```python
from build123d import *

# Parameters (mm, degrees)
BOSS_EXTRUDE1_DEPTH = 3.175
FILLET1_R           = 2
FILLET2_R           = 2
FILLET3_R           = 2


with BuildPart() as part:
    # Sketch2 → Boss-Extrude1 (new body)
    with BuildSketch(Plane(origin=(0, 0, 0), x_dir=(1, 0, 0), z_dir=(0, 1, 0))):
        with BuildLine():
            Line((0, 0), (40, 0))
            Line((40, 0), (40, 10))
            ThreePointArc((40, 10), (32.396249588, 7.141230333), (25, 10.500557105))
            Line((25, 10.500557105), (25, 20.002146828))
            Line((25, 20.002146828), (24.05, 20.002146828))
            Line((24.05, 20.002146828), (24.05, 5.002146828))
            Line((24.05, 5.002146828), (15.95, 5.002146828))
            Line((15.95, 5.002146828), (15.95, 20.002146828))
            Line((15.95, 20.002146828), (15, 20.002146828))
            Line((15, 20.002146828), (15, 9.499442895))
            ThreePointArc((15, 9.499442895), (7.396249588, 6.640673228), (0, 10))
            Line((0, 10), (0, 0))
        make_face()
    extrude(amount=BOSS_EXTRUDE1_DEPTH)

    # Fillet1
    fillet1_edges = [part.edges().sort_by_distance(p)[0] for p in [
        (15, 1.5875, -9.499442895),
        (25, 1.5875, -10.500557105),
    ]]
    fillet(fillet1_edges, radius=FILLET1_R)

    # Fillet2
    # the kernel refuses this fillet: 2 mm, written as the material it takes off along each edge
    with BuildSketch(Plane(origin=(25, -4.255511133, -20.002146828), x_dir=(0, 0, 1), z_dir=(0, 1, 0))) as fillet2_piece_1:
        with BuildLine():
            CenterArc((1.702204453, -2), FILLET2_R, 90, 58.331756746)
            Line((0, -0.95), (-0.034044089, -0.929))
            ThreePointArc((-0.034044089, -0.929), (-0.04, -0.475), (-0.04, 0))
            Line((-0.04, 0), (0, 0.04))
            Line((0, 0.04), (1.702204453, 0.04))
            Line((1.702204453, 0.04), (1.702204453, 0))
        make_face()
    extrude(amount=11.686022265, mode=Mode.SUBTRACT)
    with BuildSketch(Plane(origin=(15, -4.255511133, -20.002146828), x_dir=(0, 0, 1), z_dir=(0, 1, 0))) as fillet2_piece_2:
        with BuildLine():
            CenterArc((1.702204453, 2), FILLET2_R, 211.668243254, 58.331756746)
            Line((0, 0.95), (-0.034044089, 0.929))
            ThreePointArc((-0.034044089, 0.929), (-0.04, 0.475), (-0.04, 0))
            Line((-0.04, 0), (0, -0.04))
            Line((0, -0.04), (1.702204453, -0.04))
            Line((1.702204453, -0.04), (1.702204453, 0))
        make_face()
    extrude(amount=11.686022265, mode=Mode.SUBTRACT)
    with BuildSketch(Plane(origin=(0, -9.943835684, -10), x_dir=(0, 0, 1), z_dir=(0, 1, 0))) as fillet2_piece_3:
        with BuildLine():
            CenterArc((3.977534274, 2), FILLET2_R, 152.863608887, 117.136391113)
            Line((2.197687698, 2.912220459), (2.162090766, 2.930464868))
            ThreePointArc((2.162090766, 2.930464868), (1.193071422, 1.385002021), (-0.027308932, 0.02922708))
            Line((-0.027308932, 0.02922708), (0, -0.04))
            Line((0, -0.04), (3.977534274, -0.04))
            Line((3.977534274, -0.04), (3.977534274, 0))
        make_face()
    extrude(amount=23.062671369, mode=Mode.SUBTRACT)
    with BuildSketch(Plane(origin=(40, -9.298695448, -10), x_dir=(-0.8303470474110474, 0, 0.5572466068588987), z_dir=(0, 1, 0))) as fillet2_piece_4:
        with BuildLine():
            CenterArc((3.733360689, 1.97396451), FILLET2_R, 146.134404681, 114.610566722)
            Line((2.072666595, 3.088457724), (2.039452713, 3.110747588))
            Line((2.039452713, 3.110747588), (-0.033213882, 0.022289864))
            Line((-0.033213882, 0.022289864), (0.006433168, -0.03947929))
            ThreePointArc((0.006433168, -0.03947929), (1.705851155, 0.098074035), (3.405269143, -0.03947929))
            Line((3.405269143, -0.03947929), (3.411702311, 0))
        make_face()
    extrude(amount=21.772390895, mode=Mode.SUBTRACT)

    # Fillet3
    fillet3_edges = [part.edges().sort_by_distance(p)[0] for p in [
        (40, 1.5875, 0),
        (0, 1.5875, 0),
    ]]
    fillet(fillet3_edges, radius=FILLET3_R)


solid = part.part
```
The listing builds one solid part. Answer for the finished solid, in the listing's coordinates (mm). A direction names the side the tool comes from. Round coordinates to 2 decimals unless told otherwise and drop trailing zeros. Loops run counter-clockwise (first coordinate to the right, second up) from the corner with the lowest first, then second, coordinate; pieces in that order, holes last.
Q1. Which of the six approach directions +Z, -Z, +X, -X, +Y, -Y give full straight-line access (tool end or side, diameter ignored) to faces 1 (the face through (15, 2, -14)), 2 (the face through (20, 2, 0)), 3 (the face through (25, 2, -15)), 4 (the face through (15.95, 2, -12)), 5 (the face through (0, 2, -4))?
Q2. Section A-A, the plane z = -17 is taken. Determine the outline of the cut face in (x, y) (3 decimals).
Q3. Section B-B, the plane y = 0.95 is taken. Determine the outline of the cut face in (x, z).
Q4. Section C-C, the plane x = 18.5 is taken. Determine the outline of the cut face in (y, z) (3 decimals), then the cut area to 3 significant figures.
Q5. Given pin 1 Ø1 at (y, z) = (1.5, -15.5) entering from -X; pin 2 Ø1.6 at (x, y) = (19.5, 2) entering from -Z; pin 3 Ø4 at (x, z) = (7.5, -9) entering from +Y; pin 4 Ø1 at (y, z) = (2, -15.5) entering from +X, each flat-ended and moving along its own axis, determine where each tip first touches the part or whether it passes through.
Q6. Section D-D, the plane x = 4.5 is taken. Determine the outline of the cut face in (y, z) (3 decimals), then the cut area to 3 significant figures.
Q7. For a pull along X with two mould halves and no side action, classify faces 6 (the face through (0.982, 1.565, -7.744)), 7 (the face through (14.8, 1.61, -9.55)), 8 (the face through (24.753, 1.565, -19.262)) as released by +X, released by -X, zero draft, split by the parting line, or undercut.
Q8. Find the intervals of material crossed by line 1 (X direction, y = 3, z = -5.25); line 2 (X direction, y = 0.2, z = -13.25); line 3 (Z direction, x = 22, y = 2.7), in increasing order.
Completed:
1. face 1: -Z, -X, +Y, -Y
1. face 2: +Z, +X, -X, +Y, -Y
1. face 3: -Z, +X, +Y, -Y
1. face 4: -Z, +Y, -Y
1. face 5: +Z, -Z, -X, +Y, -Y
2. outline: (15, 0) - (15.95, 0) - (15.95, 3.175) - (15, 3.175) - close; (24.05, 0) - (25, 0) - (25, 3.175) - (24.05, 3.175) - close
3. outline: (0, -6.02) arc R2 ccw to (2.91, -7.8) arc R10.61 cw to (14.22, -8.84) arc R2 cw to (15, -10.42) - (15, -18.3) arc R2 ccw to (15.95, -20) - (15.95, -5) - (24.05, -5) - (24.05, -20) arc R2 ccw to (25, -18.3) - (25, -11.34) arc R2 cw to (25.66, -9.85) arc R10.61 cw to (37.17, -8.1) arc R2 ccw to (40, -6.28) - (40, -2) arc R2 ccw to (38, 0) - (2, 0) arc R2 ccw to (0, -2) - close
4. outline: (0, -5.002) - (3.175, -5.002) - (3.175, 0) - (0, 0) - close
4. area: 15.9 mm2
5. pin 1: stops at x = 15
5. pin 2: stops at z = -5
5. pin 3: passes through
5. pin 4: stops at x = 25
6. outline: (0, -7.145) - (3.175, -7.145) - (3.175, 0) - (0, 0) - close
6. area: 22.7 mm2
7. face 6: undercut
7. face 7: released by -X
7. face 8: released by +X
8. line 1: x = 0 to 15.95, 24.05 to 40
8. line 2: x = 15 to 15.95, 24.05 to 25
8. line 3: z = -5 to 0
